Geometry: final body of the model. Coordinates: model frame, mm. A direction names the side the tool comes from. Round coordinates to 2 decimals unless told otherwise and drop trailing zeros. Write each loop counter-clockwise with the first axis right and the second up, starting at its lowest first coordinate (ties: lowest second). Pieces come first, ordered by that corner, then holes. Notation, with made-up numbers: (45.5, 66) - (95.5, 66) arc R11 ccw to (95.5, 82) - close; hole circle Ø2 at (34.25, 88.25). An arc over 180 degrees is marked (long way). Write each question's results on one line, items separated by ' | '.
from build123d import *

# Parameters (mm, degrees)
BOSS_EXTRUDE1_DEPTH     = 28
BOSS_EXTRUDE2_DEPTH     = 10
CUT_EXTRUDE1_DEPTH      = 15.675439909
CUT_EXTRUDE1_DEPTH_BACK = 25.887131558
SKETCH3_R               = 11.5
CUT_EXTRUDE2_DEPTH      = 10
SKETCH4_R               = 1.5
CUT_EXTRUDE3_DEPTH      = 26
SKETCH5_W               = 19.5
SKETCH5_H               = 10
SKETCH5_RX              = 1.533173802
SKETCH5_RY              = 1.5
CUT_EXTRUDE4_DEPTH      = 0.6
CUT_EXTRUDE5_REACH      = 13
SKETCH6_R               = 3
CUT_EXTRUDE6_REACH      = 16
SKETCH7_R               = 3
CUT_EXTRUDE7_REACH      = 16.887
SKETCH8_R               = 1.5
CUT_EXTRUDE8_REACH      = 13.387
SKETCH9_R               = 3


with BuildPart() as part:
    # Sketch1 → Boss-Extrude1 (new body)
    with BuildSketch(Plane.XY):
        Polygon((0, 0), (49, 0), (49, 10), (-21.931026719, 25), (-24, 15.216373394), (0, 1.5), align=None)
    extrude(amount=BOSS_EXTRUDE1_DEPTH)

    # Sketch2 → Boss-Extrude2 (add)
    with BuildSketch(Plane(origin=(4.121724919, 19.490545356, 0), x_dir=(0.978362661, -0.206897328, 0), z_dir=(0.206897328, 0.978362661, 0))):
        Polygon((-13.893841917, 16), (-21.483308301, 0), (30.854721254, 0), (9.106158083, 16), align=None)
    extrude(amount=-BOSS_EXTRUDE2_DEPTH)

    # Sketch2<3> → Cut-Extrude1 (cut, two sides)
    with BuildSketch(Plane(origin=(4.121724919, 19.490545356, 0), x_dir=(0.978362661, -0.206897328, 0), z_dir=(0.206897328, 0.978362661, 0))) as cut_extrude1_sk:
        with BuildLine():
            ThreePointArc((-12.628930853, -28), (-22.528425788, -23.899494938), (-26.628930853, -14.000000004))
            Line((-26.628930853, -14.000000004), (-26.628930853, -28))
            Line((-26.628930853, -28), (-12.628930853, -28))
        make_face()
        with BuildLine():
            Line((-25.278041493, -8), (-21.483308301, 0))
            Line((-21.483308301, 0), (-26.628930853, 0))
            Line((-26.628930853, 0), (-26.628930853, -14.000000004))
            ThreePointArc((-26.628930853, -14.000000004), (-26.287033741, -10.924902359), (-25.278041493, -8))
        make_face()
    extrude(amount=CUT_EXTRUDE1_DEPTH, mode=Mode.SUBTRACT)
    extrude(cut_extrude1_sk.sketch, amount=-CUT_EXTRUDE1_DEPTH_BACK, mode=Mode.SUBTRACT)

    # Sketch3 → Cut-Extrude2 (cut)
    with BuildSketch(Plane(origin=(4.121724919, 19.490545356, 0), x_dir=(0.978362661, -0.206897328, 0), z_dir=(0.206897328, 0.978362661, 0))):
        with Locations((-12.628930853, -14)):
            Circle(SKETCH3_R)
    extrude(amount=-CUT_EXTRUDE2_DEPTH, mode=Mode.SUBTRACT)

    # Sketch4 → Cut-Extrude3 (cut, through all)
    with BuildSketch(Plane.XZ):
        with Locations((17, 8)):
            Circle(SKETCH4_R)
        with Locations((32, 8)):
            Circle(SKETCH4_R)
    extrude(amount=-CUT_EXTRUDE3_DEPTH, mode=Mode.SUBTRACT)

    # Sketch5 → Cut-Extrude4 (cut)
    with BuildSketch(Plane(origin=(4.121724919, 19.490545356, 0), x_dir=(0.978362661, -0.206897328, 0), z_dir=(0.206897328, 0.978362661, 0))):
        Polygon((-18.716315349, 0), (-3.393841917, 0), (-3.393841917, 5.75), (-15.988850867, 5.75), align=None)
        Polygon((-15.040167569, 7.75), (-3.393841917, 7.75), (-3.393841917, 13.5), (-12.312703087, 13.5), align=None)
        Polygon((-1.393841917, 7.75), (16.101510968, 7.75), (8.285621079, 13.5), (-1.393841917, 13.5), align=None)
        Polygon((20.870933117, 0), (23.870933117, 0), (26.635971254, 0), (18.820081364, 5.75), (-1.393841917, 5.75), (-1.393841917, 0), (1.370933117, 0), align=None)
        with Locations((11.120933117, -7.5)):
            Rectangle(SKETCH5_W, SKETCH5_H)
        with BuildLine():
            add(Edge.make_bspline(
                [(14.696263114, -8), (14.696263114, -5.401923789), (12.396502412, -6.700961894), (10.096741709, -8), (12.396502412, -9.299038106), (14.696263114, -10.598076211), (14.696263114, -8)],
                knots=[0, 0, 0, 2.094395102, 2.094395102, 4.188790205, 4.188790205, 6.283185307, 6.283185307, 6.283185307], degree=2, weights=[1, 0.5, 1, 0.5, 1, 0.5, 1]))
        make_face(mode=Mode.SUBTRACT)
        with Locations((11.120933117, -20.5)):
            Rectangle(SKETCH5_W, SKETCH5_H)
        with Locations((33.620933117, -20.5)):
            Rectangle(SKETCH5_W, SKETCH5_H)
        with Locations((33.620933117, -7.5)):
            Rectangle(SKETCH5_W, SKETCH5_H)
        with BuildLine():
            add(Edge.make_bspline(
                [(30.028001134, -8), (30.028001134, -5.401923789), (27.728240431, -6.700961894), (25.428479728, -8), (27.728240431, -9.299038106), (30.028001134, -10.598076211), (30.028001134, -8)],
                knots=[0, 0, 0, 2.094395102, 2.094395102, 4.188790205, 4.188790205, 6.283185307, 6.283185307, 6.283185307], degree=2, weights=[1, 0.5, 1, 0.5, 1, 0.5, 1]))
        make_face(mode=Mode.SUBTRACT)
        with Locations((13.163089313, -8)):
            Ellipse(SKETCH5_RX, SKETCH5_RY)
        with Locations((28.494827332, -8)):
            Ellipse(SKETCH5_RX, SKETCH5_RY)
    extrude(amount=-CUT_EXTRUDE4_DEPTH, mode=Mode.SUBTRACT)

    # Sketch6 → Cut-Extrude5 (cut, up to next)
    with BuildSketch(Plane(origin=(0, 14, 0), x_dir=(-1, 0, 0), z_dir=(0, -1, 0)), mode=Mode.PRIVATE) as cut_extrude5_sk1:
        with Locations((-17, -8)):
            Circle(SKETCH6_R)
    cut_extrude5_tool1 = extrude(cut_extrude5_sk1.sketch, amount=-CUT_EXTRUDE5_REACH, mode=Mode.PRIVATE) & part.part
    add(cut_extrude5_tool1.solids().sort_by_distance((17, 14, 8))[0], mode=Mode.SUBTRACT)

    # Sketch7 → Cut-Extrude6 (cut, up to next)
    with BuildSketch(Plane(origin=(0, 11, 0), x_dir=(-1, 0, 0), z_dir=(0, -1, 0)), mode=Mode.PRIVATE) as cut_extrude6_sk1:
        with Locations((-32, -8)):
            Circle(SKETCH7_R)
    cut_extrude6_tool1 = extrude(cut_extrude6_sk1.sketch, amount=-CUT_EXTRUDE6_REACH, mode=Mode.PRIVATE) & part.part
    add(cut_extrude6_tool1.solids().sort_by_distance((32, 11, 8))[0], mode=Mode.SUBTRACT)

    # Sketch8 → Cut-Extrude7 (cut, up to next)
    with BuildSketch(Plane(origin=(2.052751638, 9.70691875, 0), x_dir=(0.978362661, -0.206897328, 0), z_dir=(0.206897328, 0.978362661, 0)), mode=Mode.PRIVATE) as cut_extrude7_sk1:
        with Locations((-12.628930853, -14)):
            Circle(SKETCH8_R)
    cut_extrude7_tool1 = extrude(cut_extrude7_sk1.sketch, amount=-CUT_EXTRUDE7_REACH, mode=Mode.PRIVATE) & part.part
    add(cut_extrude7_tool1.solids().sort_by_distance((-10.302923, 12.319811, 14))[0], mode=Mode.SUBTRACT)

    # Sketch9 → Cut-Extrude8 (cut, up to next)
    with BuildSketch(Plane(origin=(1.328610989, 6.282649438, 0), x_dir=(0.978362661, -0.206897328, 0), z_dir=(0.206897328, 0.978362661, 0)), mode=Mode.PRIVATE) as cut_extrude8_sk1:
        with Locations((-12.628930853, -14)):
            Circle(SKETCH9_R)
    cut_extrude8_tool1 = extrude(cut_extrude8_sk1.sketch, amount=-CUT_EXTRUDE8_REACH, mode=Mode.PRIVATE) & part.part
    add(cut_extrude8_tool1.solids().sort_by_distance((-11.027063, 8.895541, 14))[0], mode=Mode.SUBTRACT)


solid = part.part
Q1. Section query D-D, the plane z = 20.5. Return loops of the section in (x, y).
Answer block:
outline: (-22.54, 14.38) - (0, 1.5) - (0, 0) - (49, 0) - (49, 10) - (46.55, 10.52) - (46.43, 9.93) - (27.35, 13.96) - (27.48, 14.55) - (24.54, 15.17) - (24.42, 14.59) - (5.34, 18.62) - (5.46, 19.21) - (1.05, 20.14) - (-1.02, 10.36) - (-19.58, 14.28) - (-17.52, 24.07) - (-20.37, 24.67) - close
Q2. Ray query, line 1 along Z through (x, y) = (17, 6.25); line 2 along Z through (x, y) = (39.5, 4.25); line 3 along Z through (x, y) = (17, 10.25). Return the intervals inside material, ascending.
Answer block:
line 1: 0 to 6.5, 9.5 to 28 | line 2: 0 to 28 | line 3: -12.02 to 6.5, 9.5 to 28
Q3. Mould query, pull axis X, two halves, no side actions, for faces 6 (the flat face through (-3.83, 20.56, -10.67)), 7 (the flat face through (6.279, 8.813, -6.334)), 8 (the cylindrical face through (-18.18, 19.17, 21)), 9 (the flat face through (1, 15, -16)). Classes: pulls with the +X half, pulls with the -X half, needs draft (parallel to the pull), parting line crosses it, or undercut.
Answer block:
face 6: undercut | face 7: pulls with the -X half | face 8: undercut | face 9: needs draft
Q4. Pin query (flat end, axial travel): pin 1 (2 mm diameter, centred on y = 21.5, z = 16.5, fed in from -X); pin 2 (4 mm diameter, centred on x = 14.5, z = -11, fed in from -Y); pin 3 (2.5 mm diameter, centred on x = 17, y = 17.5, fed in from -Z). Return the tip coordinate at first contact, or that it passes through.
Answer block:
pin 1: x = -22.71 | pin 2: y = 6.65 | pin 3: z = -13.88
Q5. Section query B-B, the plane z = -11. Return loops of the section in (x, y), plus the area to 3 significant figures.
Answer block:
outline: (-13.86, 13.07) - (17.61, 6.42) - (19.68, 16.2) - (15.55, 17.07) - (15.43, 16.49) - (2.63, 19.19) - (2.76, 19.78) - (0.8, 20.19) - (0.68, 19.61) - (-9.21, 21.7) - (-9.08, 22.28) - (-11.79, 22.86) - close | area: 308 mm2
Q6. Section query C-C, the plane x = 7. Return loops of the section in (y, z), plus the area to 3 significant figures.
Answer block:
outline: (0, 0) - (8.66, 0) - (8.66, -16) - (18.88, -16) - (18.88, -13.5) - (18.27, -13.5) - (18.27, -7.75) - (18.88, -7.75) - (18.88, -5.75) - (18.27, -5.75) - (18.27, 0) - (18.88, 0) - (18.88, 2.5) - (18.27, 2.5) - (18.27, 12.5) - (18.88, 12.5) - (18.88, 15.5) - (18.27, 15.5) - (18.27, 25.5) - (18.88, 25.5) - (18.88, 28) - (0, 28) - close | area: 673 mm2
Q7. Access query for faces 1 (the flat face through (24, 0, 14)), 2 (the flat face through (-12.898, 22.787, -2.915)), 3 (the flat face through (-12.168, 8.454, 10.693)), 4 (the flat face through (-9.764, 8.628, 15.291)), 5 (the flat face through (26.4, 14.5, -2.8)). Directions: +Z, -Z, +X, -X, +Y, -Y. A direction counts if a zero-diameter tool reaches every point of the face in a straight line with its end or side. Return the directions, or none.
Answer block:
face 1: +Z, -Z, +X, -X, -Y | face 2: +X | face 3: +Z, -Z, -X, -Y | face 4: none | face 5: +Y
